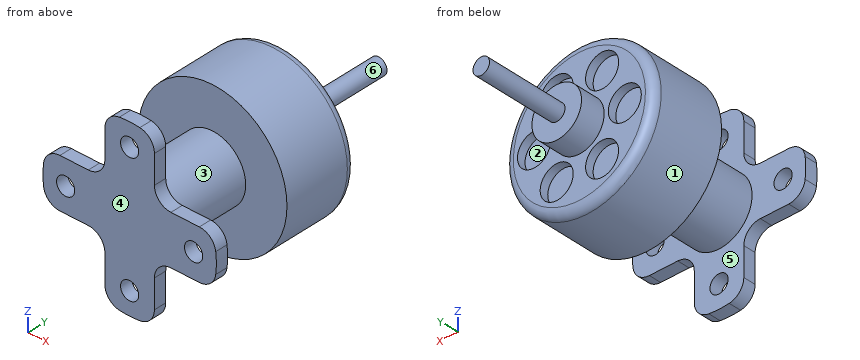
```python
from build123d import *

# Parameters (mm, degrees)
RESSALTO_EXTRUS_O1_DEPTH = 1.5
CORTE_EXTRUS_O1_REACH    = 16.925
ESBO_O2_R                = 1.1
FILETE1_R                = 2
ESBO_O3_R                = 4
RESSALTO_EXTRUS_O2_DEPTH = 9.5
ESBO_O4_R                = 9
RESSALTO_EXTRUS_O3_DEPTH = 9
FILETE2_R                = 1
ESBO_O5_R                = 3
RESSALTO_EXTRUS_O4_DEPTH = 3
ESBO_O6_R                = 1
RESSALTO_EXTRUS_O5_DEPTH = 10
ESBO_O7_R                = 2
CORTE_EXTRUS_O2_DEPTH    = 1


with BuildPart() as part:
    # Esboço1 → Ressalto-extrusão1 (new body)
    with BuildSketch(Plane(origin=(0, 0, 0), x_dir=(1, 0, 0), z_dir=(0, 1, 0))):
        with BuildLine():
            Line((-3, 3), (-3, 10.062305899))
            ThreePointArc((-3, 10.062305899), (0, 10.5), (3, 10.062305899))
            Line((3, 10.062305899), (3, 3))
            Line((3, 3), (10.062305899, 3))
            ThreePointArc((10.062305899, 3), (10.5, 0), (10.062305899, -3))
            Line((10.062305899, -3), (3, -3))
            Line((3, -3), (3, -10.062305899))
            ThreePointArc((3, -10.062305899), (0, -10.5), (-3, -10.062305899))
            Line((-3, -10.062305899), (-3, -3))
            Line((-3, -3), (-10.062305899, -3))
            ThreePointArc((-10.062305899, -3), (-10.5, 0), (-10.062305899, 3))
            Line((-10.062305899, 3), (-3, 3))
        make_face()
    extrude(amount=RESSALTO_EXTRUS_O1_DEPTH)

    # Esboço2 → Corte-extrusão1 (cut, up to next)
    with BuildSketch(Plane(origin=(0, 1.5, 0), x_dir=(1, 0, 0), z_dir=(0, 1, 0)), mode=Mode.PRIVATE) as corte_extrus_o1_sk1:
        with Locations(Location((-7.75, 0, 0), (0, 0, 270))):
            Circle(ESBO_O2_R)
    corte_extrus_o1_tool1 = extrude(corte_extrus_o1_sk1.sketch, amount=-CORTE_EXTRUS_O1_REACH, mode=Mode.PRIVATE) & part.part
    # Esboço2 → Corte-extrusão1 (cut, up to next)
    with BuildSketch(Plane(origin=(0, 1.5, 0), x_dir=(1, 0, 0), z_dir=(0, 1, 0)), mode=Mode.PRIVATE) as corte_extrus_o1_sk2:
        with Locations(Location((0, 7.75, 0), (0, 0, 270))):
            Circle(ESBO_O2_R)
    corte_extrus_o1_tool2 = extrude(corte_extrus_o1_sk2.sketch, amount=-CORTE_EXTRUS_O1_REACH, mode=Mode.PRIVATE) & part.part
    # Esboço2 → Corte-extrusão1 (cut, up to next)
    with BuildSketch(Plane(origin=(0, 1.5, 0), x_dir=(1, 0, 0), z_dir=(0, 1, 0)), mode=Mode.PRIVATE) as corte_extrus_o1_sk3:
        with Locations(Location((7.75, 0, 0), (0, 0, 270))):
            Circle(ESBO_O2_R)
    corte_extrus_o1_tool3 = extrude(corte_extrus_o1_sk3.sketch, amount=-CORTE_EXTRUS_O1_REACH, mode=Mode.PRIVATE) & part.part
    # Esboço2 → Corte-extrusão1 (cut, up to next)
    with BuildSketch(Plane(origin=(0, 1.5, 0), x_dir=(1, 0, 0), z_dir=(0, 1, 0)), mode=Mode.PRIVATE) as corte_extrus_o1_sk4:
        with Locations(Location((0, -7.75, 0), (0, 0, 270))):
            Circle(ESBO_O2_R)
    corte_extrus_o1_tool4 = extrude(corte_extrus_o1_sk4.sketch, amount=-CORTE_EXTRUS_O1_REACH, mode=Mode.PRIVATE) & part.part
    add(corte_extrus_o1_tool1.solids().sort_by_distance((-7.75, 1.5, 0))[0], mode=Mode.SUBTRACT)
    add(corte_extrus_o1_tool2.solids().sort_by_distance((0, 1.5, -7.75))[0], mode=Mode.SUBTRACT)
    add(corte_extrus_o1_tool3.solids().sort_by_distance((7.75, 1.5, 0))[0], mode=Mode.SUBTRACT)
    add(corte_extrus_o1_tool4.solids().sort_by_distance((0, 1.5, 7.75))[0], mode=Mode.SUBTRACT)

    # Filete1
    filete1_edges = [part.edges().sort_by_distance(p)[0] for p in [
        (10.062305899, 0.75, 3),
        (3, 0.75, 3),
        (3, 0.75, 10.062305899),
        (-3, 0.75, 10.062305899),
        (-3, 0.75, 3),
        (-10.062305899, 0.75, 3),
        (-10.062305899, 0.75, -3),
        (-3, 0.75, -3),
        (-3, 0.75, -10.062305899),
        (3, 0.75, -10.062305899),
        (3, 0.75, -3),
        (10.062305899, 0.75, -3),
    ]]
    fillet(filete1_edges, radius=FILETE1_R)

    # Esboço3 → Ressalto-extrusão2 (add)
    with BuildSketch(Plane(origin=(0, 1.5, 0), x_dir=(1, 0, 0), z_dir=(0, 1, 0))):
        with Locations(Location((0, 0, 0), (0, 0, 270))):
            Circle(ESBO_O3_R)
    extrude(amount=RESSALTO_EXTRUS_O2_DEPTH)

    # Esboço4 → Ressalto-extrusão3 (add)
    with BuildSketch(Plane(origin=(0, 11, 0), x_dir=(1, 0, 0), z_dir=(0, 1, 0))):
        with Locations(Location((0, 0, 0), (0, 0, 270))):
            Circle(ESBO_O4_R)
    extrude(amount=RESSALTO_EXTRUS_O3_DEPTH)

    # Filete2
    filete2_edges = [part.edges().sort_by_distance(p)[0] for p in [
        (0, 20, -9),
    ]]
    fillet(filete2_edges, radius=FILETE2_R)

    # Esboço5 → Ressalto-extrusão4 (add)
    with BuildSketch(Plane(origin=(0, 20, 0), x_dir=(1, 0, 0), z_dir=(0, 1, 0))):
        with Locations(Location((0, 0, 0), (0, 0, 270))):
            Circle(ESBO_O5_R)
    extrude(amount=RESSALTO_EXTRUS_O4_DEPTH)

    # Esboço6 → Ressalto-extrusão5 (add)
    with BuildSketch(Plane(origin=(0, 23, 0), x_dir=(1, 0, 0), z_dir=(0, 1, 0))):
        with Locations(Location((0, 0, 0), (0, 0, 270))):
            Circle(ESBO_O6_R)
    extrude(amount=RESSALTO_EXTRUS_O5_DEPTH)

    # Esboço7 → Corte-extrusão2 (cut)
    with BuildSketch(Plane(origin=(0, 20, 0), x_dir=(1, 0, 0), z_dir=(0, 1, 0))):
        with Locations(Location((-5.5, 0, 0), (0, 0, 270))):
            Circle(ESBO_O7_R)
        with Locations(Location((-2.75, 4.763139721, 0), (0, 0, 270))):
            Circle(ESBO_O7_R)
        with Locations(Location((2.75, 4.763139721, 0), (0, 0, 270))):
            Circle(ESBO_O7_R)
        with Locations(Location((5.5, 0, 0), (0, 0, 270))):
            Circle(ESBO_O7_R)
        with Locations(Location((2.75, -4.763139721, 0), (0, 0, 270))):
            Circle(ESBO_O7_R)
        with Locations(Location((-2.75, -4.763139721, 0), (0, 0, 270))):
            Circle(ESBO_O7_R)
    extrude(amount=-CORTE_EXTRUS_O2_DEPTH, mode=Mode.SUBTRACT)


solid = part.part
```
Verification items for the finished model (mm, model axes). Face numbers are marked on the shaded views. A direction names the side the tool comes from. Give positions to 0.01 mm unless a question says otherwise; leave off trailing zeros. Order: outer loops, then holes, each group sorted by start corner. A loop starts at its lowest first (then second) coordinate and runs counter-clockwise, first axis right, second up. Notation, with made-up numbers: (-6, -27) -> (20, -27) arc R9 cw to (20, -21) -> close; hole circle Ø9 at (31, 83.5). An arc over 180 degrees is marked (long way). One line per item, written item: value.
(1) Sectioned sample at B-B on y = 25. Record the cut outline in (x, z).
Final values:
outline: circle Ø2 at (0, 0)
(2) Tool access check on the marked faces 4, 5 and 6. Record the directions out of +Z, -Z, +X, -X, +Y, -Y that give a thin tool (end or side, any length) a straight path to the whole face; none if there is none.
Final values:
face 4: +Z, -Z, +X, -X, -Y
face 5: none
face 6: +Y
(3) Sectioned sample at D-D on y = 15. Record the cut outline in (x, z), then the cut area to 3 significant figures.
Final values:
outline: circle Ø18 at (0, 0)
area: 254 mm^2
(4) Gauge pin test, flat ends, axial feed: pin 1 (6 mm diameter, centred on x = -4.5, z = -0.5, fed in from +Y); pin 2 (0.8 mm diameter, centred on y = 1, z = 7, fed in from +X); pin 3 (4 mm diameter, centred on y = 14, z = 2.5, fed in from -X). Record the tip position at first contact, or that the pin passes through.
Final values:
pin 1: y = 23
pin 2: x = 3
pin 3: x = -8.99
(5) Draft check along Y on the marked faces 1, 2 and 3. Enter one of: pulls with the +Y half, pulls with the -Y half, needs draft (parallel to the pull), parting line crosses it, or undercut.
Final values:
face 1: needs draft
face 2: pulls with the +Y half
face 3: undercut
(6) Scan lines: line 1 along Y through (x, z) = (4.25, -2.75); line 2 along Y through (x, z) = (-2, 4.75); line 3 along Y through (x, z) = (9.75, -1.25). Record each from-to range of solid material in increasing order. Write a range as [from, to].
Final values:
line 1: [0, 1.5], [11, 20]
line 2: [0, 1.5], [11, 19]
line 3: [0, 1.5]
(7) Sectioned sample at A-A on z = 0. Count the separate pieces of the cut face and the enclosed holes in it, then the cut area to 3 significant figures.
Final values:
separate pieces: 3
enclosed holes: 0
area: 292 mm^2
